Autodesk Inventor part; units mm, degrees
ref_plane "YZ Plane" through (0, 0, 0) normal (1, 0, 0) x (0, 1, 0)
ref_plane "XZ Plane" through (0, 0, 0) normal (0, 1, 0) x (-1, 0, 0)
ref_plane "XY Plane" through (0, 0, 0) normal (0, 0, 1) x (1, 0, 0)
sketch "Sketch1" plane through (0, 0, 0) normal (0, 0, 1) x (1, 0, 0)
  line L0 (0, 0) -> (38.5, 0)
  line L1 (38.5, 0) -> (38.5, -80.7)
  line L2 (38.5, -80.7) -> (0, -80.7)
  line L3 (0, -80.7) -> (0, 0)
  circle A0 centre (36, -2.5) radius 1.6
  circle A1 centre (36, -78.2) radius 1.6
  dimension "d0" = 38.5
  dimension "d1" = 80.7
  dimension "d4" = 3.2
  dimension "d7" = 3.2
extrude "Extrusion1" add sketch "Sketch1" along normal blind 1
sketch "Sketch2" plane through (0, 0, 0) normal (0, 0, -1) x (-1, 0, 0)
  line L0 (0, -80.7) -> (-38.5, -80.7)
  line L1 (0, 0) -> (0, -80.7)
  line L2 (-38.5, 0) -> (0, 0)
  line L3 (-38.5, -80.7) -> (-38.5, 0)
  circle A0 centre (-36, -78.2) radius 1.6
  circle A1 centre (-36, -2.5) radius 1.6
  line L4 (-26.0363, 0) -> (-26.0363, -34.7)
  dimension "d10" = 34.7
properties part number "alert"
Source: CAD feature listing. Evaluate the final solid. Frame: model axes, mm. Give positions to 0.01 mm unless a question says otherwise; leave off trailing zeros. Order: outer loops, then holes, each group sorted by start corner. A loop starts at its lowest first (then second) coordinate and runs counter-clockwise, first axis right, second up.
(1) Material intervals for line 1 along Y through (x, z) = (36, 0.6); line 2 along X through (y, z) = (-78.2, 0.55), sorted ascending.
(2) Pull-direction query (Y, two-part tool) for faces 1 (the face through (19, -40, 0)), 2 (the face through (35.792, -79.786, 0.493)); classes: +Y half, -Y half, draft (parallel to the pull), parting line (faces both ways), or undercut.
(3) Contact query for a flat-ended pin moving along its axis: P1, Ø2.5, axis at x = 36, y = -2.5, coming from the +Z side. Output: stop coordinate, or through.
(4) Section query A-A (x = 36). Return the cut outline in (y, z), plus the area to 3 significant figures.
(5) Section query B-B (y = -2.5). Return the cut outline in (x, z).
Outcome:
1. line 1: y = -80.7 to -79.8, -76.6 to -4.1, -0.9 to 0
1. line 2: x = 0 to 34.4, 37.6 to 38.5
2. face 1: draft
2. face 2: undercut
3. P1: passes through
4. outline: (-80.7, 0) - (-79.8, 0) - (-79.8, 1) - (-80.7, 1) - close; (-76.6, 0) - (-4.1, 0) - (-4.1, 1) - (-76.6, 1) - close; (-0.9, 0) - (0, 0) - (0, 1) - (-0.9, 1) - close
4. area: 74.3 mm2
5. outline: (0, 0) - (34.4, 0) - (34.4, 1) - (0, 1) - close; (37.6, 0) - (38.5, 0) - (38.5, 1) - (37.6, 1) - close
